```python
from build123d import *

# Parameters (mm, degrees)
F0_R      = 47.5
F0_R_2    = 2.5
F0_R_3    = 9
F1_DEPTH  = 4
F0_R_4    = 52.5
F2_DEPTH  = 22
F3_DEPTH  = 25
F5_R      = 12.8477395495
F6_DEPTH  = 3
F8_DEPTH  = 3
F9_R      = 5
F9_R_2    = 2.5
F10_DEPTH = 21
F4_R      = 2.5
F11_DEPTH = 30
F14_D     = 5
F14_DEPTH = 10
F14_START = 0.2595577
F14_TIP   = 1.5021515476


with BuildPart() as f1:
    # F0 (on Top) → F1 (new body)
    with BuildSketch(Plane.XY):
        Circle(F0_R)
        with Locations((-38, 0)):
            Circle(F0_R_2, mode=Mode.SUBTRACT)
        Circle(F0_R_3, mode=Mode.SUBTRACT)
        with Locations((38, 0)):
            Circle(F0_R_2, mode=Mode.SUBTRACT)
    extrude(amount=F1_DEPTH)

    # F0 (on Top) → F2 (join)
    with BuildSketch(Plane.XY):
        Circle(F0_R_4)
        Circle(F0_R, mode=Mode.SUBTRACT)
    extrude(amount=F2_DEPTH)

    # F0 (on Top) → F3 (join)
    with BuildSketch(Plane.XY):
        Circle(F0_R_4)
        Circle(F0_R, mode=Mode.SUBTRACT)
    extrude(amount=F3_DEPTH)

    # F5 (on face) → F6 (cut)
    with BuildSketch(Plane(origin=(0, 0, 0), x_dir=(1, 0, 0), z_dir=(0, 0, -1))):
        Circle(F5_R)
    extrude(amount=-F6_DEPTH, mode=Mode.SUBTRACT)

    # F7 (on face) → F8 (cut)
    with BuildSketch(Plane(origin=(0, 0, 0), x_dir=(1, 0, 0), z_dir=(0, 0, -1))):
        Polygon((37.3229600728, -4.5689112784), (41.6182732711, -2.8707894156), (42.2953131984, 1.6981218628), (38.6770399272, 4.5689112784), (34.3817267289, 2.8707894156), (33.7046868016, -1.6981218628), align=None)
        Polygon((-40.3094010768, -4), (-35.6905989232, -4), (-33.3811978465, 0), (-35.6905989232, 4), (-40.3094010768, 4), (-42.6188021535, 0), align=None)
    extrude(amount=-F8_DEPTH, mode=Mode.SUBTRACT)

    # F9 (on face) → F10 (join)
    with BuildSketch(Plane.XY.offset(4)):
        with Locations((38, 0)):
            Circle(F9_R)
        with Locations((38, 0)):
            Circle(F9_R_2, mode=Mode.SUBTRACT)
        with Locations((-38, 0)):
            Circle(F9_R)
        with Locations((-38, 0)):
            Circle(F9_R_2, mode=Mode.SUBTRACT)
        with Locations((38, 0)):
            Circle(F9_R_2)
        with Locations((-38, 0)):
            Circle(F9_R_2)
    extrude(amount=F10_DEPTH)

    # F4 (on face) → F11 (cut)
    with BuildSketch(Plane(origin=(0, 0, 0), x_dir=(1, 0, 0), z_dir=(0, 0, -1))):
        with Locations((-38, 0)):
            Circle(F4_R)
        with Locations((38, 0)):
            Circle(F4_R)
    extrude(amount=-F11_DEPTH, mode=Mode.SUBTRACT)

    # F14
    # its depths count from where the whole tool has entered the part; down to there all is cleared
    with Locations(Plane.XZ.offset(52.7).offset(-F14_START)):
        with Locations((0, 9.7180558369)):
            Hole(F14_D / 2, depth=F14_DEPTH)
            with Locations((0, 0, -(F14_DEPTH + F14_TIP / 2))):  # 118° drill point
                Cone(0, F14_D / 2, F14_TIP, mode=Mode.SUBTRACT)


solid = f1.part
```
The listing builds one solid part. Answer for the finished solid, in the listing's coordinates (mm). A direction names the side the tool comes from. Give positions to 0.01 mm unless a question says otherwise; leave off trailing zeros. Order: outer loops, then holes, each group sorted by start corner. A loop starts at its lowest first (then second) coordinate and runs counter-clockwise, first axis right, second up. Notation, with made-up numbers: M 16,32 L 28,32 A17 ccw 28,53 Z; hole C 9.25,52.5 d8. An arc over 180 degrees is marked long. Put each result on its own line as item: value. Start each with the question number.
Item 1: Flat-ended cylindrical pins translate along their axes: P1, Ø2.5, axis at x = -39.5, y = 1.5, coming from the -Z side; P2, Ø1, axis at x = 7.5, y = 34.5, coming from the +Z side; P3, Ø1, axis at y = 34, z = 20.5, coming from the +X side; P4, Ø6, axis at x = 17, y = -1, coming from the -Z side. Find the tip coordinate at first contact, or state that the pin passes through.
Item 2: Find the intervals of material crossed by line 1 along Y through (x, z) = (35, 9.75); line 2 along Y through (x, z) = (38, 11.25) (3 decimals); line 3 along Y through (x, z) = (42, 17.25), in increasing order.
Item 3: Which of the six approach directions +Z, -Z, +X, -X, +Y, -Y give full straight-line access (tool end or side, diameter ignored) to faces 4 (the face through (-35.69, 0.96, 13.85)), 5 (the face through (11, -11, 0)), 6 (the face through (33, 0, 14)), 7 (the face through (0.3, -49.9, 12.2)), 8 (the face through (-10.196, 7.818, 1.479))?
Item 4: The part is cut by section C-C, the plane x = -38. Determine the outline of the cut face in (y, z) (3 decimals).
Item 5: For a pull along X with two mould halves and no side action, classify faces 1 (the face through (50.076, 15.77, 12.325)), 2 (the face through (40.31, 0.96, 13.85)), 3 (the face through (-36, -2, 25)) as +X half, -X half, draft (parallel to the pull), parting line (faces both ways), or undercut.
Item 6: The part is cut by section D-D, the plane y = 7. Determine the outline of the cut face in (x, z).
Item 7: The part is cut by section A-A, the plane x = 0. Determine the outline of the cut face in (y, z).
Item 8: The part is cut by section B-B, the plane z = 19.75. Determine the outline of the cut face in (x, y), and give its area (3 significant figures).
Answer key:
1. P1: stops at z = 3
1. P2: stops at z = 4
1. P3: stops at x = 40.42
1. P4: stops at z = 0
2. line 1: y = -39.13 to -32.11, -4 to 4, 32.11 to 39.13
2. line 2: y = -36.225 to -28.5, -5 to -2.5, 2.5 to 5, 28.5 to 36.225
2. line 3: y = -31.5 to -22.19, -3 to 3, 22.19 to 31.5
3. face 4: +Z, -Z
3. face 5: -Z, +X, -X, +Y, -Y
3. face 6: +Z
3. face 7: -Y
3. face 8: -Z
4. outline: M -36.225,0 L -4,0 L -4,3 L -2.5,3 L -2.5,25 L -5,25 L -5,4 L -28.5,4 L -28.5,25 L -36.225,25 Z; M 2.5,3 L 4,3 L 4,0 L 36.225,0 L 36.225,25 L 28.5,25 L 28.5,4 L 5,4 L 5,25 L 2.5,25 Z
5. face 1: parting line
5. face 2: undercut
5. face 3: draft
6. outline: M -52.03,0 L -10.77,0 L -10.77,3 L -5.66,3 L -5.66,4 L -46.98,4 L -46.98,25 L -52.03,25 Z; M 5.66,3 L 10.77,3 L 10.77,0 L 52.03,0 L 52.03,25 L 46.98,25 L 46.98,4 L 5.66,4 Z
7. outline: M -52.5,0 L -12.85,0 L -12.85,3 L -9,3 L -9,4 L -47.5,4 L -47.5,7.22 L -52.5,7.22 Z; M -52.5,12.22 L -47.5,12.22 L -47.5,25 L -52.5,25 Z; M 9,3 L 12.85,3 L 12.85,0 L 52.5,0 L 52.5,25 L 47.5,25 L 47.5,4 L 9,4 Z
8. outline: C 0,0 d105; C -38,0 d10; C 38,0 d10; hole C 0,0 d95; hole C -38,0 d5; hole C 38,0 d5
8. area: 1,690 mm²
